Verification items for this drawing (mm, ordinates from the low corner). A direction names the side the tool comes from. Give positions to 0.01 mm unless a question says otherwise; leave off trailing zeros. Order: outer loops, then holes, each group sorted by start corner. A loop starts at its lowest first (then second) coordinate and runs counter-clockwise, first axis right, second up. Notation, with made-up numbers: M -6.5,31.5 L 39.5,31.5 A27 cw 39.5,70.5 Z; hole C 18,16 d7. An arc over 180 degrees is marked long. One line per question, with ' | ' between items. Start each with the question number.
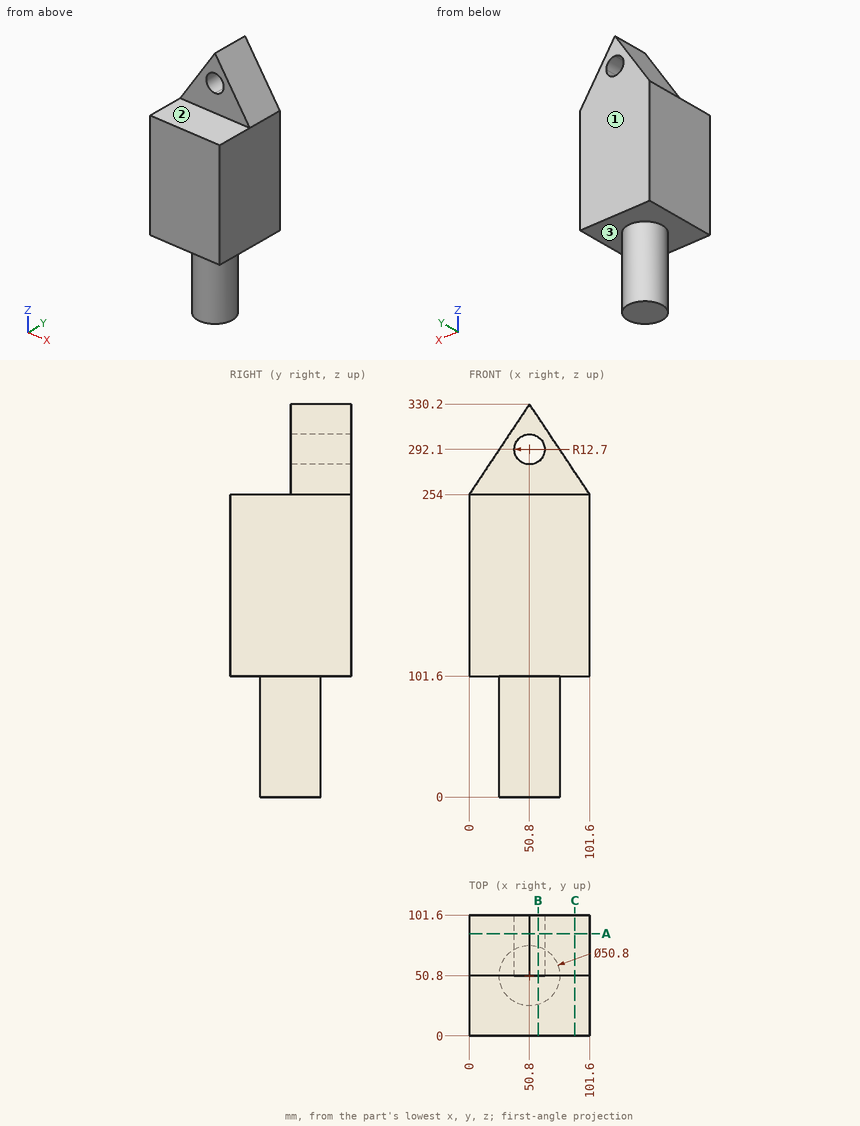
Item 1: Depth check by flat-ended pin: pin 1 (5 mm diameter, centred on y = 69, z = 202.5, fed in from -X); pin 2 (6 mm diameter, centred on x = 11, y = 18, fed in from -Z); pin 3 (4 mm diameter, centred on x = 14, y = 33.5, fed in from +Z). Enter the tip coordinate at first touch or a pass-through.
Item 2: Cross-section at B-B, the plane x = 58. Record the cut outline in (y, z), plus the area to 3 significant figures.
Item 3: Material ranges on line 1 along Y through (x, z) = (47, 256); line 2 along Z through (x, y) = (11, 4); line 3 along Z through (x, y) = (46.5, 88.5), recorded low to high.
Item 4: Cross-section at C-C, the plane x = 89. Record the cut outline in (y, z).
Item 5: Cross-section at A-A, the plane y = 86. Record the cut outline in (x, z).
Item 6: Set-up check for the marked faces 1, 2 and 3: record each of +Z, -Z, +X, -X, +Y, -Y from which the full face is reachable in a straight line by a thin tool's end or side.
Outcome:
1) pin 1: stops at x = 0 | pin 2: stops at z = 101.6 | pin 3: stops at z = 254
2) outline: M 0,101.6 L 26.44,101.6 L 26.44,0 L 75.16,0 L 75.16,101.6 L 101.6,101.6 L 101.6,281.64 L 50.8,281.64 L 50.8,254 L 0,254 Z; M 50.8,302.56 L 101.6,302.56 L 101.6,319.4 L 50.8,319.4 Z | area: 22,700 mm²
3) line 1: y = 50.8 to 101.6 | line 2: z = 101.6 to 254 | line 3: z = 101.6 to 280.15, 304.05 to 323.75
4) outline: M 0,101.6 L 101.6,101.6 L 101.6,272.9 L 50.8,272.9 L 50.8,254 L 0,254 Z
5) outline: M 0,101.6 L 101.6,101.6 L 101.6,254 L 50.8,330.2 L 0,254 Z; hole M 50.8,304.8 A12.7 ccw long 63.5,292.1 A12.7 ccw Z
6) face 1: +Z, -Z, +X, -X, +Y | face 2: +Z, +X, -X, -Y | face 3: -Z
